Autodesk Inventor part; units mm, degrees
ref_plane "YZ Plane" through (0, 0, 0) normal (1, 0, 0) x (0, 1, 0)
ref_plane "XZ Plane" through (0, 0, 0) normal (0, 1, 0) x (-1, 0, 0)
ref_plane "XY Plane" through (0, 0, 0) normal (0, 0, 1) x (1, 0, 0)
sketch "Sketch9" plane through (0, 0, 0) normal (0, 1, 0) x (-1, 0, 0)
  line L0 (15, 15) -> (-15, 15)
  line L1 (-15, 15) -> (-15, -15)
  line L2 (-15, -15) -> (15, -15)
  line L3 (15, -15) -> (15, 15)
  line L4 (15, 15) -> (-15, -15) construction
  line L5 (-15, 15) -> (15, -15) construction
  line L6 (-13, 13) -> (13, 13)
  line L7 (13, 13) -> (13, -13)
  line L8 (13, -13) -> (-13, -13)
  line L9 (-13, -13) -> (-13, 13)
  point P0 (0, 0)
  dimension "d172" = 30
  dimension "d173" = 30
  dimension "d174" = 2
extrude "Extrusion3" add sketch "Sketch9" against normal blind 405
sketch "Sketch10" plane through (0, 0, 0) normal (1, 0, 0) x (0, 1, 0)
  line L0 (0, 15) -> (0, -15) construction
  line L1 (0, 15) -> (-405, 15) construction
  line L2 (-405, -15) -> (-405, 15) construction
  line L3 (0, -15) -> (-405, -15) construction
  line L4 (-68.5, 8.5) -> (-51.5, 8.5)
  line L5 (-51.5, 8.5) -> (-51.5, -8.5)
  line L6 (-51.5, -8.5) -> (-68.5, -8.5)
  line L7 (-68.5, -8.5) -> (-68.5, 8.5)
  line L8 (-68.5, 8.5) -> (-51.5, -8.5) construction
  line L9 (-51.5, 8.5) -> (-68.5, -8.5) construction
  line L10 (0, 0) -> (30, 0)
  circle A0 centre (-60, 0) radius 8.5
  dimension "d177" = 17
  dimension "d178" = 17
  dimension "d181" = 30
  dimension "d182" = 90
extrude "Extrusion4" cut sketch "Sketch10" along normal through all contours A0
pattern_linear "Rectangular Pattern4" count 4 spacing 85 along (0, -1, 0) of "Extrusion4"
properties part number "PRS 8661 FDS 1000 way tube 1_940" material "Stainless Steel"
The listing builds one solid part. Answer for the finished solid, in the listing's coordinates (mm). A direction names the side the tool comes from. Give positions to 0.01 mm unless a question says otherwise; leave off trailing zeros. Write each loop counter-clockwise with the first axis right and the second up, starting at its lowest first coordinate (ties: lowest second). Pieces come first, ordered by that corner, then holes. Notation, with made-up numbers: (77.5, 83.25) - (112.5, 83.25) arc R16 ccw to (112.5, 112.25) - close; hole circle Ø5 at (-4.75, 42). An arc over 180 degrees is marked (long way). Use one line per item in the form item = value. Start each with the question number.
1) Consider line 1 along Y through (x, z) = (13.65, 0); line 2 along Z through (x, y) = (-6.5, -25); line 3 along Z through (x, y) = (13.6, -315). Determine where each line is inside the solid, lowest interval first. Write a range as from..to.
2) Find section C-C on y = -345.5. Determine the outline of the cut face in (x, z), plus the area to 3 significant figures.
3) Find section D-D on y = -230. Determine the outline of the cut face in (x, z), plus the area to 3 significant figures.
4) A tool of negligible diameter and unlimited length cuts with its end or side. For faces 4 (the face through (0, -200, 15)), 5 (the face through (-13, -200, 0)), 6 (the face through (13.99, -323.49, -0.37)), from which of +Z, -Z, +X, -X, +Y, -Y can it reach the whole face along a straight path? Write none if from no direction.
5) A flat-ended cylindrical pin translates along its axis: pin 1 Ø6 at (x, z) = (-8.5, -8) entering from +Y. Find the tip coordinate at first contact, or state that the pin passes through.
6) Find section A-A on z = 0. Determine the outline of the cut face in (x, y), plus the area to 3 significant figures.
7) The mould has two halves that part along Y. Classify faces 1 (the face through (13.99, -136.89, -2.55)), 2 (the face through (0, -200, 13)), 3 (the face through (14, -405, 0)): pulls with the +Y half, pulls with the -Y half, needs draft (parallel to the pull), parting line crosses it, or undercut.
8) Find section B-B on x = -1. Determine the outline of the cut face in (y, z).
Geometry results:
q1.line_1 = -405..-323.5, -306.5..-238.5, -221.5..-153.5, -136.5..-68.5, -51.5..0
q1.line_2 = -15..-13, 13..15
q1.line_3 = -15..-8.5, 8.5..15
q2.outline = (-15, -15) - (15, -15) - (15, 15) - (-15, 15) - close; hole (-13, -13) - (13, -13) - (13, 13) - (-13, 13) - close
q2.area = 224 mm2
q3.outline = (-15, -15) - (15, -15) - (15, -8.5) - (13, -8.5) - (13, -13) - (-13, -13) - (-13, 13) - (13, 13) - (13, 8.5) - (15, 8.5) - (15, 15) - (-15, 15) - close
q3.area = 190 mm2
q4.face_4 = +Z, +X, -X, +Y, -Y
q4.face_5 = +Y, -Y
q4.face_6 = +X
q5.pin_1 = through
q6.outline = (-15, -405) - (-13, -405) - (-13, 0) - (-15, 0) - close; (13, -405) - (15, -405) - (15, -323.5) - (13, -323.5) - close; (13, -306.5) - (15, -306.5) - (15, -238.5) - (13, -238.5) - close; (13, -221.5) - (15, -221.5) - (15, -153.5) - (13, -153.5) - close; (13, -136.5) - (15, -136.5) - (15, -68.5) - (13, -68.5) - close; (13, -51.5) - (15, -51.5) - (15, 0) - (13, 0) - close
q6.area = 1,480 mm2
q7.face_1 = undercut
q7.face_2 = needs draft
q7.face_3 = pulls with the -Y half
q8.outline = (-405, -15) - (0, -15) - (0, -13) - (-405, -13) - close; (-405, 13) - (0, 13) - (0, 15) - (-405, 15) - close
